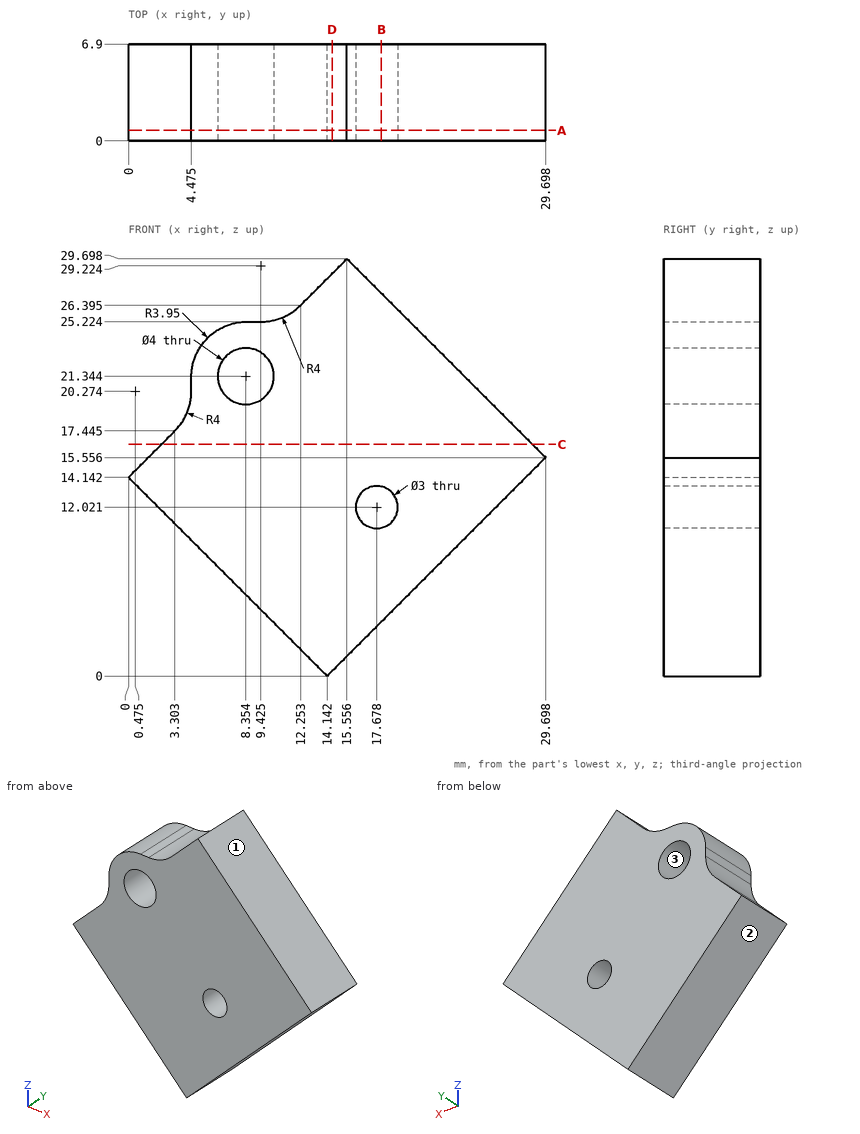
Here's the drawing with two shaded views (mm, measured from the low corner). I have some questions. Give positions to 0.01 mm unless a question says otherwise; leave off trailing zeros. Order: outer loops, then holes, each group sorted by start corner. A loop starts at its lowest first (then second) coordinate and runs counter-clockwise, first axis right, second up.
Q1. We'd pull the mould along X, two halves only. Please class the marked faces 1, 2 and 3: +X half, -X half, draft (parallel to the pull), parting line (faces both ways), or undercut.
Q2. Suppose I cut it at A-A, the plane y = 0.75. Count the separate pieces of the cut face and the enclosed holes in it.
Q3. Suppose I cut it at B-B, the plane x = 18. Write out the boundary of the cut face in (y, z) (1 decimal), and give its area (3 significant figures).
Q4. If I drill on line 1 along Z through (x, y) = (7.5, 0.5) (1 decimal); line 2 along Z through (x, y) = (18.75, 4.5) (1 decimal); line 3 along X through (y, z) = (5, 5.75) (1 decimal), over which ranges is the centre line in solid material (lowest first)?
Q5. Suppose I cut it at C-C, the plane z = 16.5. Write out the boundary of the cut face in (x, y) (1 decimal).
Q6. I'm going to push flat-ended pins straight in: P1, Ø1.1, axis at x = 9, y = 5, coming from the +Z side; P2, Ø6, axis at x = 26.5, z = 4.5, coming from the +Y side; P3, Ø2, axis at x = 26, y = 2.5, coming from the +Z side (1 decimal); P4, Ø0.8, axis at y = 2.5, z = 21, coming from the -X side (1 decimal). Where does each tip first touch, or does it pass through?
Q7. Suppose I cut it at D-D, the plane x = 14.5. Write out the boundary of the cut face in (y, z), and give its area (3 significant figures).
Solution:
1. face 1: +X half
1. face 2: -X half
1. face 3: undercut
2. separate pieces: 1
2. enclosed holes: 2
3. outline: (0, 3.9) - (6.9, 3.9) - (6.9, 10.6) - (0, 10.6) - close; (0, 13.5) - (6.9, 13.5) - (6.9, 27.3) - (0, 27.3) - close
3. area: 141 mm2
4. line 1: z = 6.6 to 19.5, 23.2 to 25.1
4. line 2: z = 4.6 to 11, 13.1 to 26.5
4. line 3: x = 8.4 to 19.9
5. outline: (2.4, 0) - (28.8, 0) - (28.8, 6.9) - (2.4, 6.9) - close
6. P1: stops at z = 25.23
6. P2: passes through
6. P3: stops at z = 20.3
6. P4: stops at x = 4.5
7. outline: (0, 0.36) - (6.9, 0.36) - (6.9, 28.64) - (0, 28.64) - close
7. area: 195 mm2
